Can you work these out from the model? Positions are in its coordinate system, mm. Face numbers are marked on the shaded views. A direction names the side the tool comes from. Round coordinates to 2 decimals unless told otherwise and drop trailing zeros. Order: outer loops, then holes, each group sorted by start corner. A loop starts at its lowest first (then second) coordinate and runs counter-clockwise, first axis right, second up.
Q1. If we section it at A-A (z = -0.25): Please give me the cut outline in (x, y), plus the area to 3 significant figures.
Q2. Will these pins go through, and if not, where does the flat tip stop? P1, Ø3, axis at x = 0, z = -2.5, coming from the -Y side; P2, Ø1, axis at x = -0.5, y = -2, coming from the -Z side; P3, Ø1, axis at x = -1.5, z = -3, coming from the -Y side.
Q3. We'd pull the mould along X, two halves only. Please class the marked faces 4, 5 and 6: pulls with the +X half, pulls with the -X half, needs draft (parallel to the pull), parting line crosses it, or undercut.
Q4. For the marked faces 1, 2 and 3, which set-ups out of +Z, -Z, +X, -X, +Y, -Y let a thin tool reach every point of the face, with its end or its side?
Q5. If I drill on line 1 (Z direction, x = -2.1, y = -1); line 2 (X direction, y = -0.75, z = -1.5); line 3 (Y direction, x = 0.1, z = 0.5), over which ranges is the centre line in solid material (lowest first)?
Autodesk Inventor part; units mm, degrees
ref_plane "YZ Plane" through (0, 0, 0) normal (1, 0, 0) x (0, 1, 0)
ref_plane "XZ Plane" through (0, 0, 0) normal (0, 1, 0) x (-1, 0, 0)
ref_plane "XY Plane" through (0, 0, 0) normal (0, 0, 1) x (1, 0, 0)
sketch "スケッチ1" plane through (0, 0, 0) normal (0, 0, 1) x (1, 0, 0)
  circle A0 centre (0, 0) radius 2.55
  dimension "d0" = 5.1
extrude "押し出し1" add sketch "スケッチ1" along normal blind 1.2
sketch "スケッチ2" plane through (0, 0, 0) normal (0, 0, -1) x (-1, 0, 0)
  circle A0 centre (0, 0) radius 2.55
  circle A1 centre (0, 0) radius 1.5
  dimension "d3" = 3
extrude "押し出し2" add sketch "スケッチ2" along normal blind 6 contours A1
thread "ねじ1"
sketch "スケッチ3" plane through (0, 0, 1.2) normal (0, 0, 1) x (1, 0, 0)
  circle A0 centre (0, 0) radius 2.55
  line L0 (0, 1.1547) -> (1, 0.5774)
  line L1 (1, 0.5774) -> (1, -0.5774)
  line L2 (1, -0.5774) -> (0, -1.1547)
  line L3 (0, -1.1547) -> (-1, -0.5774)
  line L4 (-1, -0.5774) -> (-1, 0.5774)
  line L5 (-1, 0.5774) -> (0, 1.1547)
  dimension "d8" = 2
extrude "押し出し3" cut sketch "スケッチ3" against normal blind 1 contours L0 L1 L2 L3 L4 L5
fillet "フィレット1" radius 0.2 2 edges at (-2.55, 0, 1.2) (-2.55, 0, 0)
chamfer "面取り1" distance 0.2 angle 45 1 edges at (1.5, 0, -6)
properties part number "六角穴付低頭平 M3 x 6" material "鋼"
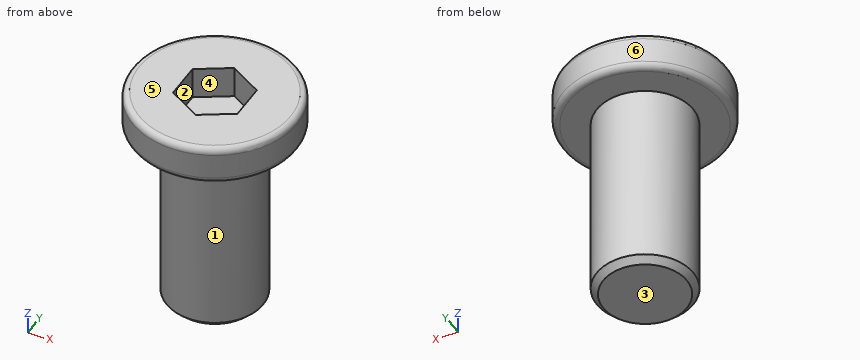
Solution:
1. outline: circle Ø3 at (0, 0)
1. area: 7.07 mm2
2. P1: stops at y = -1.5
2. P2: stops at z = 0
2. P3: stops at y = -1.12
3. face 4: undercut
3. face 5: needs draft
3. face 6: parting line crosses it
4. face 1: -Z
4. face 2: +Z
4. face 3: -Z, +X, -X, +Y, -Y
5. line 1: z = 0 to 1.2
5. line 2: x = -1.3 to 1.3
5. line 3: y = -2.55 to -1.1, 1.1 to 2.55
